Part model, mm, in its own coordinate system. A direction names the side the tool comes from. Give positions to 0.01 mm unless a question says otherwise; leave off trailing zeros. Write each loop counter-clockwise with the first axis right and the second up, starting at its lowest first coordinate (ties: lowest second). Pieces come first, ordered by that corner, then holes.
Autodesk Inventor part; units mm, degrees
ref_plane "YZ Plane" through (0, 0, 0) normal (1, 0, 0) x (0, 1, 0)
ref_plane "XZ Plane" through (0, 0, 0) normal (0, 1, 0) x (-1, 0, 0)
ref_plane "XY Plane" through (0, 0, 0) normal (0, 0, 1) x (1, 0, 0)
sketch "Sketch1" plane through (0, 0, 0) normal (0, 1, 0) x (-1, 0, 0)
  line L0 (37, 0) -> (0, 0)
  line L1 (0, 0) -> (-3.25, -15)
  line L2 (-3.25, -15) -> (3.25, -15)
  line L3 (3.25, -15) -> (3.25, -8.5)
  line L4 (3.25, -8.5) -> (33.75, -8.5)
  line L5 (33.75, -8.5) -> (33.75, -15)
  line L6 (33.75, -15) -> (40.25, -15)
  line L7 (40.25, -15) -> (37, 0)
  line L8 (37, 0) -> (47, 0)
  line L9 (47, 0) -> (47, -20)
  line L10 (47, -20) -> (-10, -20)
  line L11 (-10, -20) -> (-10, 0)
  line L12 (-10, 0) -> (0, 0)
  dimension "d1" = 20
  dimension "d5" = 10
  dimension "d6" = 10
extrude "Extrusion1" add sketch "Sketch1" along normal blind 300 contours L8 L9 L10 L11 L12 L1 L2 L3 L4 L5 L6 L7
sketch "Sketch2" plane through (10, 0, -20) normal (0, 0, -1) x (-1, 0, 0)
  line L0 (0, 0) -> (57, 0)
  line L1 (57, 0) -> (57, 300)
  line L2 (0, 300) -> (57, 300)
  line L3 (0, 0) -> (0, 300)
  line L4 (43.75, 0) -> (13.25, 0)
  line L5 (28.5, 0) -> (28.5, 300)
  line L6 (43.75, 300) -> (13.25, 300)
  line L7 (0, 52.5) -> (57, 52.5)
  line L8 (57, 52.5) -> (57, 247.5)
  line L9 (57, 247.5) -> (0, 247.5)
  line L10 (0, 247.5) -> (0, 52.5)
  line L11 (0, 52.5) -> (57, 247.5) construction
  line L12 (57, 52.5) -> (0, 247.5) construction
  circle A0 centre (28.5, 150) radius 3.1
  line L13 (28.5, 52.5) -> (28.5, 82.5)
  circle A1 centre (28.5, 82.5) radius 3.1
  line L14 (28.5, 247.5) -> (28.5, 217.5)
  circle A2 centre (28.5, 217.5) radius 3.1
  point P0 (10, 0)
  dimension "d7" = 195
  dimension "d8" = 6.2
  dimension "d9" = 30
  dimension "d10" = 6.2
  dimension "d11" = 30
  dimension "d12" = 6.2
extrude "Extrusion2" cut sketch "Sketch2" against normal up to surface (11.5 mm away) contours A1 L5 | L5 A1 | A2 L5 | L5 A2 | A0 L5 | L5 A0
sketch "Sketch4" plane through (-33.75, 0, -8.5) normal (0, 0, 1) x (1, 0, 0)
  circle A0 centre (15.25, 217.5) radius 3.1
  circle A1 centre (15.25, 82.5) radius 3.1
  circle A2 centre (15.25, 150) radius 3.1
  line L0 (0, 0) -> (30.5, 0)
  line L1 (30.5, 0) -> (30.5, 300)
  line L2 (0, 300) -> (30.5, 300)
  line L3 (0, 0) -> (0, 300)
  circle A3 centre (15.25, 82.5) radius 3.1
  circle A4 centre (15.25, 82.5) radius 5
  circle A5 centre (15.25, 150) radius 5
  circle A6 centre (15.25, 217.5) radius 5
  point P0 (33.75, 0)
  dimension "d15" = 10
  dimension "d16" = 10
  dimension "d17" = 10
extrude "Extrusion3" cut sketch "Sketch4" against normal blind 6 contours A4 | A5 | A6
properties part number "uchwyt_szyny"
1) 3-axis set-ups, long thin cutter, end or side, ignore diameter. For faces 1 (the face through (-19.151, 222.457, -11.458)), 2 (the face through (-33.75, 148, -12)), 3 (the face through (-37, 148, -15)), 4 (the face through (-17.828, 214.474, -17.288)): which of +Z, -Z, +X, -X, +Y, -Y reach the whole face in a straight line?
Answers follow:
face 1: +Z
face 2: +Z, +Y, -Y
face 3: +Y, -Y
face 4: +Z, -Z
2) Pin check, flat tips, straight feed: pin 1 Ø8 at (x, y) = (-18.5, 217.5) entering from +Z; pin 2 Ø8 at (x, y) = (-17.5, 219) entering from +Z; pin 3 Ø12 at (x, z) = (-18.5, -10.5) entering from -Y; pin 4 Ø5.5 at (x, y) = (-18.5, 217.5) entering from -Z. Stop position of each tip, or through.
Answers follow:
pin 1: stops at z = -14.5
pin 2: stops at z = -8.5
pin 3: stops at y = 0
pin 4: passes through
3) Two-plate mould, pull along X, no slides. Class faces 5 (the face through (-13, 148, -20)), 6 (the face through (-38.648, 147.9, -7.605)), 7 (the face through (10, 148, -10)): +X half, -X half, draft (parallel to the pull), parting line (faces both ways), or undercut.
Answers follow:
face 5: draft
face 6: undercut
face 7: +X half
4) Saw through at C-C, the plane z = -5.5. Write the cut outline in (x, y), then the cut area to 4 significant figures.
Answers follow:
outline: (-47, 0) - (-38.19, 0) - (-38.19, 300) - (-47, 300) - close; (1.19, 0) - (10, 0) - (10, 300) - (1.19, 300) - close
area: 5,285 mm2
5) Saw through at A-A, the plane x = -18.5. Write the cut outline in (y, z), then the cut area to 3 significant figures.
Answers follow:
outline: (0, -20) - (79.4, -20) - (79.4, -14.5) - (77.5, -14.5) - (77.5, -8.5) - (0, -8.5) - close; (85.6, -20) - (146.9, -20) - (146.9, -14.5) - (145, -14.5) - (145, -8.5) - (87.5, -8.5) - (87.5, -14.5) - (85.6, -14.5) - close; (153.1, -20) - (214.4, -20) - (214.4, -14.5) - (212.5, -14.5) - (212.5, -8.5) - (155, -8.5) - (155, -14.5) - (153.1, -14.5) - close; (220.6, -20) - (300, -20) - (300, -8.5) - (222.5, -8.5) - (222.5, -14.5) - (220.6, -14.5) - close
area: 3,170 mm2
6) Wall check: L1, parallel to Y at x = -18.5, z = -10.55; L2, parallel to Y at x = -18.5, z = -17.1; L3, parallel to X at y = 150, z = -16.2. Give the ranges that are in metal, low to high.
Answers follow:
L1: y = 0 to 77.5, 87.5 to 145, 155 to 212.5, 222.5 to 300
L2: y = 0 to 79.4, 85.6 to 146.9, 153.1 to 214.4, 220.6 to 300
L3: x = -47 to -21.6, -15.4 to 10
7) Saw through at D-D, the plane y = 196.5. Write the cut outline in (x, z), then the cut area to 4 significant figures.
Answers follow:
outline: (-47, -20) - (10, -20) - (10, 0) - (0, 0) - (3.25, -15) - (-3.25, -15) - (-3.25, -8.5) - (-33.75, -8.5) - (-33.75, -15) - (-40.25, -15) - (-37, 0) - (-47, 0) - close
area: 734.5 mm2
8) Saw through at B-B, the plane y = 82.5. Write the cut outline in (x, z).
Answers follow:
outline: (-47, -20) - (-21.6, -20) - (-21.6, -14.5) - (-23.5, -14.5) - (-23.5, -8.5) - (-33.75, -8.5) - (-33.75, -15) - (-40.25, -15) - (-37, 0) - (-47, 0) - close; (-15.4, -20) - (10, -20) - (10, 0) - (0, 0) - (3.25, -15) - (-3.25, -15) - (-3.25, -8.5) - (-13.5, -8.5) - (-13.5, -14.5) - (-15.4, -14.5) - close
